Work out the finished part from the listing and answer in its coordinate system (mm). Face numbers are marked on the shaded views. Give positions to 0.01 mm unless a question says otherwise; leave off trailing zeros. Loops run counter-clockwise (first coordinate to the right, second up) from the corner with the lowest first, then second, coordinate; pieces in that order, holes last. Notation, with made-up numbers: (-37.75, 57) - (7.25, 57) arc R23 ccw to (7.25, 83) - close; hole circle Ø6 at (-9, 28.5). An arc over 180 degrees is marked (long way). One line per question, with ' | ' between items.
from build123d import *

# Parameters (mm, degrees)
SKETCH_1_W      = 10
SKETCH_1_H      = 10
SKETCH_1_R      = 1.5
EXTRUDE_1_DEPTH = 5
SKETCH_2_R      = 1
EXTRUDE_2_DEPTH = 5


with BuildPart() as part:
    # 草图1 → 凸台-拉伸1 (new body)
    with BuildSketch(Plane(origin=(0, 0, 0), x_dir=(1, 0, 0), z_dir=(0, 1, 0))):
        with Locations((5, 5)):
            Rectangle(SKETCH_1_W, SKETCH_1_H)
        with Locations(Location((7.5, 7.5, 0), (0, 0, 270))):
            Circle(SKETCH_1_R, mode=Mode.SUBTRACT)
        with Locations(Location((7.5, 2.5, 0), (0, 0, 270))):
            Circle(SKETCH_1_R, mode=Mode.SUBTRACT)
        with Locations(Location((4, 7.5, 0), (0, 0, 270))):
            Circle(SKETCH_1_R, mode=Mode.SUBTRACT)
    extrude(amount=EXTRUDE_1_DEPTH)

    # 草图2 → 凸台-拉伸2 (add)
    with BuildSketch(Plane(origin=(0, 0, -10), x_dir=(-1, 0, 0), z_dir=(0, 0, -1))):
        with Locations((-5, 2.5)):
            Circle(SKETCH_2_R)
    extrude(amount=EXTRUDE_2_DEPTH)


solid = part.part
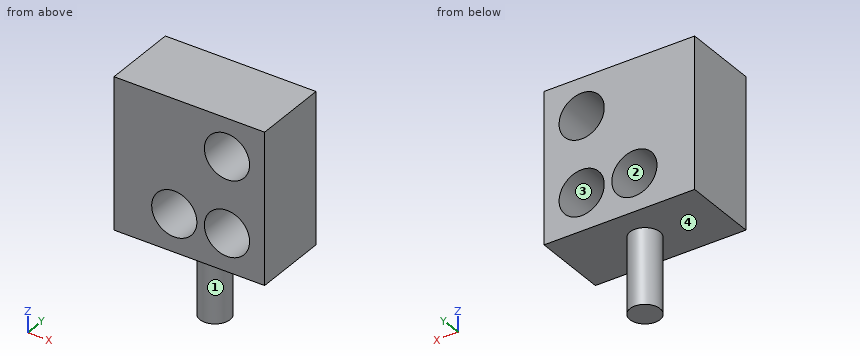
1. Find section D-D on x = 5. Write down the section's boundary in (y, z).
Evaluation:
outline: (0, -10) - (1.5, -10) - (1.5, -15) - (3.5, -15) - (3.5, -10) - (5, -10) - (5, -8.62) - (0, -8.62) - close; (0, -6.38) - (5, -6.38) - (5, 0) - (0, 0) - close
2. Determine the mould class of the marked faces 1, 2, 3 and 4 for opening direction Z: +Z half, -Z half, draft (parallel to the pull), parting line (faces both ways), or undercut.
Evaluation:
face 1: draft | face 2: undercut | face 3: undercut | face 4: -Z half
3. Flat-ended cylindrical pins translate along their axes: pin 1 (2 mm diameter, centred on x = 1.5, y = 3.5, fed in from -Z); pin 2 (3 mm diameter, centred on x = 7, z = -11, fed in from -Y); pin 3 (2.5 mm diameter, centred on x = 7.5, z = -2.5, fed in from -Y). Find the tip coordinate at first contact, or state that the pin passes through.
Evaluation:
pin 1: z = -10 | pin 2: y = 0 | pin 3: through
4. Consider L1, parallel to X at y = 2.55, z = -7.5; L2, parallel to X at y = 3, z = -2.5; L3, parallel to Z at x = 6.5, y = 2. Determine where each line is inside the solid, lowest interval first.
Evaluation:
L1: 0 to 2.5, 5.5 to 6, 9 to 10 | L2: 0 to 6, 9 to 10 | L3: -10 to -8.62, -6.38 to -3.62, -1.38 to 0
5. Find section B-B on z = -7.5. Write down the section's boundary in (x, y), then the cut area to 3 significant figures.
Evaluation:
outline: (0, 0) - (2.5, 0) - (2.5, 5) - (0, 5) - close; (5.5, 0) - (6, 0) - (6, 5) - (5.5, 5) - close; (9, 0) - (10, 0) - (10, 5) - (9, 5) - close | area: 20.0 mm2
6. Find section C-C on x = 7.5. Write down the section's boundary in (y, z).
Evaluation:
outline: (0, -10) - (5, -10) - (5, -9) - (0, -9) - close; (0, -6) - (5, -6) - (5, -4) - (0, -4) - close; (0, -1) - (5, -1) - (5, 0) - (0, 0) - close
7. Find section A-A on y = 0.8. Write down the section's boundary in (x, z), then the cut area to 3 significant figures.
Evaluation:
outline: (0, -10) - (10, -10) - (10, 0) - (0, 0) - close; hole circle Ø3 at (4, -7.5); hole circle Ø3 at (7.5, -7.5); hole circle Ø3 at (7.5, -2.5) | area: 78.8 mm2
